Geometry check sheet. Reference: the model listing, model coordinates, mm. Coordinates: 2 decimals unless noted, no trailing zeros. Write each loop counter-clockwise with the first axis right and the second up, starting at its lowest first coordinate (ties: lowest second). Pieces come first, ordered by that corner, then holes.
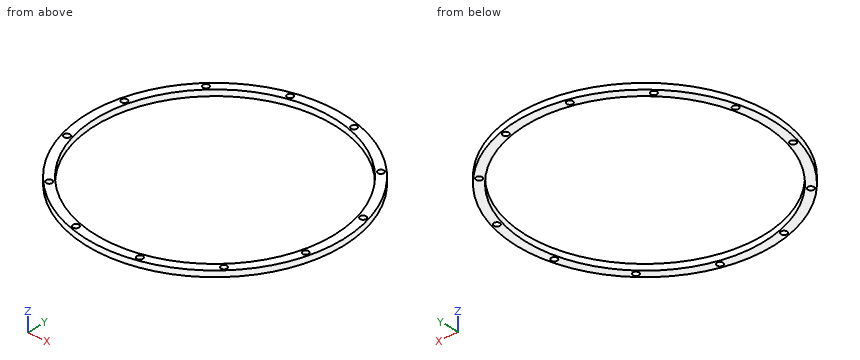
from build123d import *

# Parameters (mm, degrees)
FLANGESKETCH_R      = 546.101092202
FLANGESKETCH_R_2    = 508.001016002
FLANGEFEATURE_DEPTH = 25.4000508
SKETCH2_R           = 12.7
BOLT_HOLE_DEPTH     = 26.4000508
BOLTPATTERN_COUNT   = 12


with BuildPart() as part:
    # FlangeSketch → FlangeFeature (new body)
    with BuildSketch(Plane.XY):
        Circle(FLANGESKETCH_R)
        Circle(FLANGESKETCH_R_2, mode=Mode.SUBTRACT)
    extrude(amount=FLANGEFEATURE_DEPTH)

    # Sketch2 → Bolt Hole (cut, through all)
    with BuildSketch(Plane.XY.offset(25.4000508)):
        with Locations((-136.410860404, 509.092261732)):
            Circle(SKETCH2_R)
    bolt_hole = extrude(amount=-BOLT_HOLE_DEPTH, mode=Mode.SUBTRACT)

    # BoltPattern: Bolt Hole ×12 about axis
    boltpattern_axis = Axis((0, 0, 0), (0, 0, 1))
    for i in range(1, BOLTPATTERN_COUNT):
        add(bolt_hole.rotate(boltpattern_axis, i * 360 / BOLTPATTERN_COUNT), mode=Mode.SUBTRACT)


solid = part.part
1. Sectioned sample at A-A, the plane y = 0. Record the boundary of the cut face in (x, z), and give its area (3 significant figures).
Computed values:
outline: (-546.1, 0) - (-508, 0) - (-508, 25.4) - (-546.1, 25.4) - close; (508, 0) - (546.1, 0) - (546.1, 25.4) - (508, 25.4) - close
area: 1,940 mm2
2. Sectioned sample at C-C, the plane z = 12.25. Give the number of separate pieces and of enclosed holes in the cut face, and give its area (3 significant figures).
Computed values:
separate pieces: 1
enclosed holes: 13
area: 120,000 mm2
3. Thickness scan on line 1 along Y through (x, z) = (0, 11); line 2 along X through (y, z) = (390, 6.75); line 3 along Y through (x, z) = (367.5, 24.25). Record the ranges inside material, lowest first.
Computed values:
line 1: y = -546.1 to -508, 508 to 546.1
line 2: x = -382.26 to -325.52, 325.52 to 382.26
line 3: y = -403.94 to -384.28, -361.09 to -350.73, 350.73 to 361.09, 384.28 to 403.94
4. Gauge pin test, flat ends, axial feed: pin 1 Ø1 at (x, z) = (429.5, 16.5) entering from -Y; pin 2 Ø3 at (y, z) = (74.5, 8.5) entering from +X; pin 3 Ø2 at (y, z) = (317, 11) entering from +X. Record the tip position at first contact, or that the pin passes through.
Computed values:
pin 1: stops at y = -337.91
pin 2: stops at x = 541.2
pin 3: stops at x = 445.39
